Build history of the part. All positions in model axes, mm. A direction names the side the tool comes from. Round coordinates to 2 decimals unless told otherwise and drop trailing zeros. Loops run counter-clockwise (first coordinate to the right, second up) from the corner with the lowest first, then second, coordinate; pieces in that order, holes last. Notation, with made-up numbers: (-35, 15.25) - (-10, 15.25) arc R20 ccw to (-10, 40.25) - close; hole circle Ø4 at (15.5, 19). An arc over 180 degrees is marked (long way). Put each result on its own line as item: value. Start each with the question number.
from build123d import *

# Parameters (mm, degrees)
CHANFREIN2_SIZE              = 1
CHANFREIN2_SIZE_2            = 1.732050808
CHANFREIN3_SIZE              = 0.5
CHANFREIN3_SIZE2             = 0.866025404
ENROULEMENT2_SECTION_W       = 0.2
ENROULEMENT2_SECTION_H       = 3.3494767
ENROULEMENT2_ANGLE           = 3.543505781
R_P_TITION_CIRCULAIRE3_COUNT = 8
CHANFREIN4_SIZE              = 0.2
CONG_1_R                     = 0.1


# Some blends are built 0.0001 mm under size
with BuildPart() as part:
    # Esquisse1 → Révolution1 (revolve)
    with BuildSketch(Plane.XY, mode=Mode.PRIVATE) as r_volution1_sk:
        Polygon((-5.844561756, 3.794871795), (-5.844561756, -2.205128205), (-7.344561756, -2.205128205), (-7.344561756, -3.205128205), (-1.844561756, -3.205128205), (-1.844561756, -2.205128205), (-4.844561756, -2.205128205), (-4.844561756, 3.794871795), align=None)
    revolve(r_volution1_sk.sketch.rotate(Axis((-1.844561756, -3.205128205, 0), (0, 1, 0)), 270), axis=Axis((-1.844561756, -3.205128205, 0), (0, 1, 0)))

    # Chanfrein2
    # the kernel refuses this chamfer: 1.732050808, 1 mm, written as the material it takes off along each edge
    with BuildSketch(Plane(origin=(-1.844561756, -3.205128205, 0), x_dir=(0, 0, -1), z_dir=(1, 0, 0))) as chanfrein2_piece_1:
        Polygon((5.5, CHANFREIN2_SIZE), (5.5 - CHANFREIN2_SIZE_2, 0), (5.5, 0), align=None)
    revolve(axis=Axis((-1.844561756, -3.205128205, 0), (0, 1, 0)), mode=Mode.SUBTRACT)

    # Chanfrein3
    chanfrein3_edges = [part.edges().sort_by_distance(p)[0] for p in [
        (-1.844561756, 3.794871795, 4),
    ]]
    chanfrein3_side = [part.faces().sort_by_distance(p)[0] for p in [
        (-1.844561756, 3.794871795, 3.113137085),
    ]]
    chamfer(chanfrein3_edges, length=CHANFREIN3_SIZE, length2=CHANFREIN3_SIZE2, reference=chanfrein3_side[0])

    # Enroulement2 section (on wrap section) → Enroulement2 (revolve)
    with BuildSketch(Plane(origin=(-1.844561756, 3.794871795, 0), x_dir=(-0.8414709848078965, 0, 0.5403023058681398), z_dir=(0.5403023058681398, 0, 0.8414709848078965))):
        with Locations((4.1, 4.32526165)):
            Rectangle(ENROULEMENT2_SECTION_W, ENROULEMENT2_SECTION_H)
    enroulement2 = revolve(axis=Axis((-1.844561756, 3.794871795, 0), (0, -1, 0)), revolution_arc=ENROULEMENT2_ANGLE)

    # Répétition circulaire3: Enroulement2 ×8 about axis
    r_p_tition_circulaire3_axis = Axis((-1.844561756, 0, 0), (0, 1, 0))
    for i in range(1, R_P_TITION_CIRCULAIRE3_COUNT):
        add(enroulement2.rotate(r_p_tition_circulaire3_axis, i * 360 / R_P_TITION_CIRCULAIRE3_COUNT))

    # Chanfrein4
    chanfrein4_edges = [part.edges().sort_by_distance(p)[0] for p in [
        (-2.865436347, 1.144348495, 4.074041614),
        (0.31435335, 1.144348495, 3.602649798),
        (2.229479857, 1.144348495, 1.020874591),
        (1.758088041, 1.144348495, -2.158915106),
        (-0.823687166, 1.144348495, -4.074041614),
        (-4.003476862, 1.144348495, -3.602649798),
        (-5.91860337, 1.144348495, -1.020874591),
        (-5.447211554, 1.144348495, 2.158915106),
    ]]
    chamfer(chanfrein4_edges, length=CHANFREIN4_SIZE - 0.0001)  # a hair under: the kernel refuses the full size

    # Congé1
    cong_1_edges = [part.edges().sort_by_distance(p)[0] for p in [
        (-2.7389871, -0.630339855, 4.103657308),
        (-2.990909484, -0.630339855, 4.04053052),
        (0.201934522, -0.630339855, 3.667676783),
        (2.195968764, -0.630339855, 1.146347728),
        (1.823115026, -0.630339855, -2.046496279),
        (-0.698214029, -0.630339855, -4.04053052),
        (-3.891058035, -0.630339855, -3.667676783),
        (-5.885092277, -0.630339855, -1.146347728),
        (-5.512238539, -0.630339855, 2.046496279),
        (-5.378739893, -0.630339855, 2.269269685),
        (-5.948219065, -0.630339855, -0.894425344),
        (-4.113831441, -0.630339855, -3.534178136),
        (-0.950136413, -0.630339855, -4.103657308),
        (1.68961638, -0.630339855, -2.269269685),
        (2.259095552, -0.630339855, 0.894425344),
        (0.424707928, -0.630339855, 3.534178136),
    ]]
    fillet(cong_1_edges, radius=CONG_1_R)


solid = part.part
1) Slice it at A-A, the plane z = 0. Write the cut outline in (x, y).
2) Pull direction Z, two halves, no side cores. Call faces 1 (the face through (-3, 3.795, 3)), 2 (the face through (0.82, 0.84, -1.38)): pulls with the +Z half, pulls with the -Z half, needs draft (parallel to the pull), parting line crosses it, or undercut.
3) Which spindle directions (+Z, -Z, +X, -X, +Y, -Y) get a long thin tool onto all of the face, cutting with end or side? Do faces 3 (the face through (-5.81, 0.33, 0.52)), 4 (the face through (-2, -3.205, 0)). Say none if no direction does.
4) Drill centre lines: line 1 (Z direction, x = -2, y = 2.25); line 2 (X direction, y = 1.55, z = 0); line 3 (Y direction, x = -3.75, z = 2). Where is each one in solid material? Low to high. Write a range as [from, to].
5) Drop flat-ended pins along their axis: pin 1 Ø5.5 at (x, z) = (-1.84, 0) entering from +Y; pin 2 Ø3 at (x, z) = (0.5, -3) entering from -Y; pin 3 Ø1.5 at (y, z) = (-1, 0) entering from -X; pin 4 Ø2 at (x, y) = (2, 0) entering from +Z. Give the stop position or say it passes through.
6) Slice it at B-B, the plane y = 2.75. Write the cut outline in (x, z).
Taken from the geometry:
1. outline: (-7.34, -2.21) - (-5.61, -3.21) - (1.92, -3.21) - (3.66, -2.21) - (2.16, -2.21) - (2.16, 2.93) - (1.66, 3.79) - (1.16, 3.79) - (1.16, -2.21) - (-4.84, -2.21) - (-4.84, 3.79) - (-5.34, 3.79) - (-5.84, 2.93) - (-5.84, -2.21) - close
2. face 1: needs draft
2. face 2: undercut
3. face 3: +Y
3. face 4: +Z, -Z, +X, -X, -Y
4. line 1: z = [-4, -3], [3, 4]
4. line 2: x = [-5.84, -4.84], [1.16, 2.16]
4. line 3: y = [-3.21, -2.21]
5. pin 1: stops at y = -2.21
5. pin 2: stops at y = -3.21
5. pin 3: stops at x = -5.84
5. pin 4: stops at z = 2.81
6. outline: circle Ø8 at (-1.84, 0); hole circle Ø6 at (-1.84, 0)
